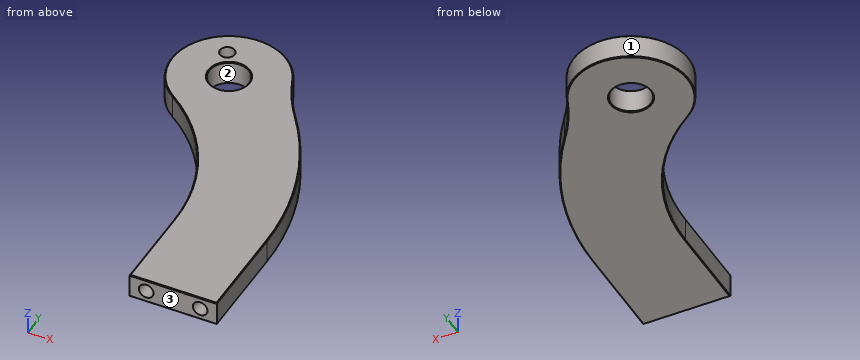
```python
from build123d import *

# Parameters (mm, degrees)
F0_R     = 8.1
F1_DEPTH = 10
F2_SIZE  = 0.3
F3_R     = 3
F4_DEPTH = 8
F5_R     = 3
F6_DEPTH = 20


with BuildPart() as f1:
    # F0 (on Top) → F1 (new body)
    with BuildSketch(Plane.XY):
        with BuildLine():
            Line((0, 36.103194), (0, 0))
            Line((0, 0), (35.6, 0))
            Line((35.6, 0), (35.6, 40))
            ThreePointArc((35.6, 40), (29.690096, 75.901135), (12.584081, 108.013479))
            ThreePointArc((12.584081, 108.013479), (6.847931, 116.701894), (2.363287, 126.097635))
            ThreePointArc((2.363287, 126.097635), (-33.971495, 135.809329), (-32.663158, 98.221809))
            ThreePointArc((-32.663158, 98.221809), (-8.663511, 71.194519), (0, 36.103194))
        make_face()
        with Locations((-19.4, 117.5)):
            Circle(F0_R, mode=Mode.SUBTRACT)
    extrude(amount=F1_DEPTH)

    # F2
    f2_edges = [f1.edges().sort_by_distance(p)[0] for p in [
        (17.8, 0, 10),
        (0, 18.051597, 10),
        (-27.5, 117.5, 10),
        (29.690096, 75.901135, 0),
        (-27.5, 117.5, 0),
        (17.8, 0, 0),
    ]]
    chamfer(f2_edges, length=F2_SIZE)

    # F3 (on face) → F4 (cut)
    with BuildSketch(Plane.XY.offset(10)):
        with Locations((-26.2, 129.5)):
            Circle(F3_R)
    extrude(amount=-F4_DEPTH, mode=Mode.SUBTRACT)

    # F5 (on face) → F6 (cut)
    with BuildSketch(Plane.XZ):
        with Locations((6.8, 5)):
            Circle(F5_R)
        with Locations((28.8, 5)):
            Circle(F5_R)
    extrude(amount=-F6_DEPTH, mode=Mode.SUBTRACT)


solid = f1.part
```
Could you check a few things on this model? Use its own coordinates, in mm. Face numbers are marked on the shaded views. Round coordinates to 2 decimals unless told otherwise and drop trailing zeros. Order: outer loops, then holes, each group sorted by start corner. A loop starts at its lowest first (then second) coordinate and runs counter-clockwise, first axis right, second up. Notation, with made-up numbers: M 55,-24 L 67,-24 A7 cw 67,-19 Z; hole C 0,89 d5. An arc over 180 degrees is marked long. One line per question, with ' | ' between items. Start each with the question number.
(1) Suppose I cut it at A-A on z = 5. List the corners of the cut face in (x, y) for me, then the cut area to 3 significant figures.
(2) For P1, Ø3, axis at x = -17.5, z = 3, coming from the -Y side; P2, Ø4, axis at x = -11.5, z = 1, coming from the +Y side; P3, Ø1.5, axis at x = -27.5, z = 3, coming from the -Y side, each with a flat end and sliding along its axis, tell me the tip position at first contact or that it passes through.
(3) Thinking about a two-plate mould opening in Y: for the marked faces 1, 2 and 3, which applies, +Y half, -Y half, draft (parallel to the pull), parting line (faces both ways), or undercut?
(4) Please list where these lines run through material, in increasing order: line 1 along X through (y, z) = (18.5, 2.5); line 2 along Y through (x, z) = (-26.2, 5.5); line 3 along Z through (x, y) = (6.8, 9.5).
Geometry results:
1) outline: M -32.66,98.22 A75.4 cw 0,36.1 L 0,0 L 3.8,0 L 3.8,20 L 9.8,20 L 9.8,0 L 25.8,0 L 25.8,20 L 31.8,20 L 31.8,0 L 35.6,0 L 35.6,40 A112 ccw 12.58,108.01 A75.4 cw 2.36,126.1 A23.4 ccw long Z; hole C -26.2,129.5 d6; hole C -19.4,117.5 d16.2 | area: 5,200 mm²
2) P1: y = 82.54 | P2: y = 140.14 | P3: y = 93.71
3) face 1: parting line | face 2: undercut | face 3: -Y half
4) line 1: 0 to 5.14, 8.46 to 27.14, 30.46 to 35.6 | line 2: 93.24 to 113.1, 121.9 to 126.5, 132.5 to 139.89 | line 3: 0 to 2, 8 to 10
